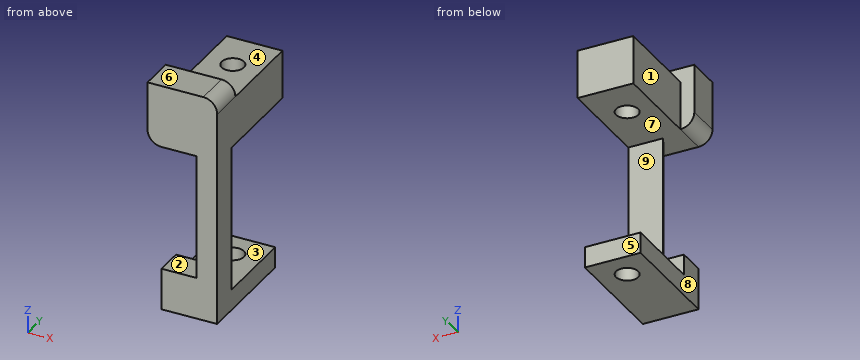
```python
from build123d import *

# Parameters (mm, degrees)
BOSS_EXTRUDE1_DEPTH = 8
CUT_EXTRUDE2_DEPTH  = 21
BOSS_EXTRUDE2_DEPTH = 3
BOSS_EXTRUDE5_DEPTH = 5
SKETCH6_R           = 1.6
CUT_EXTRUDE3_DEPTH  = 38.215588132


with BuildPart() as part:
    # Sketch1 → Boss-Extrude1 (new body)
    with BuildSketch(Plane(origin=(0, 0, 0), x_dir=(0, 0, -1), z_dir=(1, 0, 0))):
        Polygon((0, 0), (0, 16), (-3, 16), (-3, 4), (-24, 4), (-24, 18), (-31, 18), (-31, 0), align=None)
    extrude(amount=-BOSS_EXTRUDE1_DEPTH)

    # Sketch5 → Cut-Extrude2 (cut)
    with BuildSketch(Plane.XY.offset(3)):
        Polygon((-8, 0), (-3, 0), (-5, 4), (-8, 4), align=None)
    extrude(amount=CUT_EXTRUDE2_DEPTH, mode=Mode.SUBTRACT)

    # Sketch8 → Boss-Extrude2 (add)
    with BuildSketch(Plane.XY.offset(3)):
        Polygon((-8, 4), (-5, 4), (-3, 0), (-8, 0), align=None)
    extrude(amount=BOSS_EXTRUDE2_DEPTH)

    # Sketch11 → Boss-Extrude5 (add)
    with BuildSketch(Plane.XZ):
        with BuildLine():
            Line((-10, 26), (-10, 33))
            Line((-10, 33), (-2, 33))
            ThreePointArc((-2, 33), (-0.585786438, 32.414213562), (0, 31))
            Line((0, 31), (-8, 31))
            Line((-8, 31), (-8, 24))
            ThreePointArc((-8, 24), (-9.414213562, 24.585786438), (-10, 26))
        make_face()
    extrude(amount=-BOSS_EXTRUDE5_DEPTH)

    # Sketch6 → Cut-Extrude3 (cut, through all)
    with BuildSketch(Plane.XY.offset(31)):
        with Locations((-4, 12)):
            Circle(SKETCH6_R)
    extrude(amount=-CUT_EXTRUDE3_DEPTH, mode=Mode.SUBTRACT)


solid = part.part
```
CAD build for the part. Positions are in the model's coordinates, mm. Face numbers are marked on the shaded views. A direction names the side the tool comes from. Round coordinates to 2 decimals unless told otherwise and drop trailing zeros. Write each loop counter-clockwise with the first axis right and the second up, starting at its lowest first coordinate (ties: lowest second). Pieces come first, ordered by that corner, then holes. Notation, with made-up numbers: (74, 58.25) -> (121, 58.25) arc R26 cw to (121, 84.25) -> close; hole circle Ø1 at (-39, 12.25). An arc over 180 degrees is marked (long way). Answer in a Markdown table with one row per item. Add a question column.
Item 1: Which spindle directions (+Z, -Z, +X, -X, +Y, -Y) get a long thin tool onto all of the face, cutting with end or side? Do the marked faces 1, 2, 3, 4 and 5. Say none if no direction does.
Item 2: Drop flat-ended pins along their axis: pin 1 Ø4 at (x, y) = (-6, 10) entering from +Z; pin 2 Ø2.5 at (x, y) = (-4, 12) entering from -Z; pin 3 Ø4 at (x, z) = (-7.5, 25.5) entering from -Y; pin 4 Ø3 at (y, z) = (8.5, 1.5) entering from -X. Give the stop position or say it passes through.
Item 3: Saw through at C-C, the plane y = 12. Write the cut outline in (x, z), then the cut area to 3 significant figures.
Item 4: Mould opens along Z. For the marked faces 6, 7, 8 and 9 say: pulls with the +Z half, pulls with the -Z half, needs draft (parallel to the pull), parting line crosses it, or undercut.
Item 5: Saw through at B-B, the plane x = -4. Write the cut outline in (y, z), then the cut area to 3 significant figures.
Item 6: Drill centre lines: line 1 (Y direction, x = -4, z = 26.5); line 2 (Z direction, x = -7, y = 2); line 3 (Z direction, x = -3.75, y = 4.5). Where is each one in solid material? Low to high. Write a range as from..to.
Item 7: Saw through at D-D, the plane x = -6. Write the cut outline in (y, z), then the cut area to 3 significant figures.
Item 8: Saw through at A-A, the plane y = 8. Write the cut outline in (x, z), then the cut area to 3 significant figures.
Findings below:
| question | item | result |
|---|---|---|
| 1 | face 1 | +Z, -Z, -X, +Y |
| 1 | face 2 | -X, -Y |
| 1 | face 3 | +X, -X, +Y |
| 1 | face 4 | +Z, +X, -X, +Y |
| 1 | face 5 | -Z, +X, -X, +Y |
| 2 | pin 1 | stops at z = 31 |
| 2 | pin 2 | passes through |
| 2 | pin 3 | stops at y = 0 |
| 2 | pin 4 | stops at x = -8 |
| 3 | outline | (-8, 0) -> (-5.6, 0) -> (-5.6, 3) -> (-8, 3) -> close; (-8, 24) -> (-5.6, 24) -> (-5.6, 31) -> (-8, 31) -> close; (-2.4, 0) -> (0, 0) -> (0, 3) -> (-2.4, 3) -> close; (-2.4, 24) -> (0, 24) -> (0, 31) -> (-2.4, 31) -> close |
| 3 | area | 48.0 mm^2 |
| 4 | face 6 | pulls with the +Z half |
| 4 | face 7 | undercut |
| 4 | face 8 | needs draft |
| 4 | face 9 | undercut |
| 5 | outline | (0, 0) -> (10.4, 0) -> (10.4, 3) -> (4, 3) -> (4, 24) -> (10.4, 24) -> (10.4, 31) -> (5, 31) -> (5, 33) -> (0, 33) -> (0, 24) -> (2, 24) -> (2, 6) -> (0, 6) -> close; (13.6, 0) -> (16, 0) -> (16, 3) -> (13.6, 3) -> close; (13.6, 24) -> (18, 24) -> (18, 31) -> (13.6, 31) -> close |
| 5 | area | 200 mm^2 |
| 6 | line 1 | y = 0..10.4, 13.6..18 |
| 6 | line 2 | z = 0..6, 24..33 |
| 6 | line 3 | z = 0..3, 24..33 |
| 7 | outline | (0, 0) -> (16, 0) -> (16, 3) -> (4, 3) -> (4, 6) -> (0, 6) -> close; (0, 24) -> (18, 24) -> (18, 31) -> (5, 31) -> (5, 33) -> (0, 33) -> close |
| 7 | area | 196 mm^2 |
| 8 | outline | (-8, 0) -> (0, 0) -> (0, 3) -> (-8, 3) -> close; (-8, 24) -> (0, 24) -> (0, 31) -> (-8, 31) -> close |
| 8 | area | 80.0 mm^2 |
